Can you work these out from the model? Positions are in its coordinate system, mm. Give positions to 0.01 mm unless a question says otherwise; leave off trailing zeros. Loops run counter-clockwise (first coordinate to the right, second up) from the corner with the lowest first, then second, coordinate; pieces in that order, holes last.
from build123d import *

# Parameters (mm, degrees)
F1_DEPTH = 38.1


with BuildPart() as f1:
    # F0 (on Top) → F1 (new body, symmetric)
    with BuildSketch(Plane.XY):
        with BuildLine():
            ThreePointArc((-57.303448, 158.919445), (-71.415787, 118.625188), (-76.2, 76.2))
            Line((-76.2, 76.2), (-76.2, -76.2))
            ThreePointArc((-76.2, -76.2), (-71.296996, -108.039645), (-57.042274, -136.929182))
            ThreePointArc((-57.042274, -136.929182), (-34.756607, -160.191845), (-6.504878, -175.672228))
            ThreePointArc((-6.504878, -175.672228), (0, -176.817227), (6.504878, -175.672228))
            ThreePointArc((6.504878, -175.672228), (34.756607, -160.191845), (57.042274, -136.929182))
            ThreePointArc((57.042274, -136.929182), (71.296996, -108.039645), (76.2, -76.2))
            Line((76.2, -76.2), (76.2, 76.2))
            ThreePointArc((76.2, 76.2), (71.415787, 118.625188), (57.303448, 158.919445))
            ThreePointArc((57.303448, 158.919445), (37.914532, 190.746873), (12.7, 218.190317))
            ThreePointArc((12.7, 218.190317), (0, 223.041285), (-12.7, 218.190317))
            ThreePointArc((-12.7, 218.190317), (-37.914532, 190.746873), (-57.303448, 158.919445))
        make_face()
    extrude(amount=F1_DEPTH, both=True)


solid = f1.part
(1) Please list where these lines run through material, in increasing order: probe 1 along X at (y, z) = (79.5, 11.5); probe 2 along Y at (x, z) = (-45, -18.5); probe 3 along Y at (x, z) = (-22, 10.5).
Returned:
probe 1: x = -76.17 to 76.17
probe 2: y = -151.24 to 180.67
probe 3: y = -168.58 to 209.29
(2) Suppose I cut it at C-C on y = -107.5. List the corners of the cut face in (x, z) for me, plus the area to 3 significant figures.
Returned:
outline: (-71.47, -38.1) - (71.47, -38.1) - (71.47, 38.1) - (-71.47, 38.1) - close
area: 10,900 mm2
(3) Suppose I cut it at A-A on z = -9. List the corners of the cut face in (x, y) for me.
Returned:
outline: (-76.2, -76.2) arc R105.83 ccw to (-57.04, -136.93) arc R105.83 ccw to (-6.5, -175.67) arc R19.05 ccw to (6.5, -175.67) arc R105.83 ccw to (57.04, -136.93) arc R105.83 ccw to (76.2, -76.2) - (76.2, 76.2) arc R190.5 ccw to (57.3, 158.92) arc R190.5 ccw to (12.7, 218.19) arc R19.05 ccw to (-12.7, 218.19) arc R190.5 ccw to (-57.3, 158.92) arc R190.5 ccw to (-76.2, 76.2) - close
(4) Thinking about a two-plate mould opening in Z: for faces 1 (the flat face through (-1, 26, -38.1)), 2 (the flat face through (-1, 26, 38.1)), 3 (the cylindrical face through (0.19, 223.04, 0.53)), which applies, pulls with the +Z half, pulls with the -Z half, needs draft (parallel to the pull), parting line crosses it, or undercut?
Returned:
face 1: pulls with the -Z half
face 2: pulls with the +Z half
face 3: needs draft
(5) Will these pins go through, and if not, where does the flat tip stop? P1, Ø5, axis at x = 47, z = -25.5, coming from the +Y side; P2, Ø10, axis at x = 48.5, z = 11.5, coming from the -Y side; P3, Ø8, axis at y = 98, z = 16.5, coming from the -X side.
Returned:
P1: stops at y = 181.43
P2: stops at y = -152.7
P3: stops at x = -75.37
(6) Suppose I cut it at B-B on x = -43. List the corners of the cut face in (y, z) for me.
Returned:
outline: (-153.17, -38.1) - (183.66, -38.1) - (183.66, 38.1) - (-153.17, 38.1) - close
